Design review of the part built by this model. Coordinates are the model's own, in mm. A direction names the side the tool comes from. Round coordinates to 2 decimals unless told otherwise and drop trailing zeros. Order: outer loops, then holes, each group sorted by start corner. A loop starts at its lowest first (then second) coordinate and runs counter-clockwise, first axis right, second up. Notation, with made-up numbers: M 72,19.25 L 104,19.25 A32 ccw 104,52.25 Z; hole C 79,-3.75 d7. An arc over 180 degrees is marked long. Write each question's results on one line, items separated by ' | '. Start each with the question number.
Item 1: Clearance check with a flat-ended pin moving along its axis: pin 1 (1.3 mm diameter, centred on y = -2, z = 8.5, fed in from +X). State where the tip first meets the part, or that it passes through.
Item 2: Wall thickness on line 1 (Z direction, x = -31.6, y = -1.25); line 2 (X direction, y = -1.7, z = 10): over which ranges is each line inside the solid? List them lowest first. Write a range as [from, to].
Item 3: Take a section at A-A, the plane y = -1.27. Write out the cut boundary in (x, z), plus the area to 3 significant figures.
Item 4: The part is to be moulded in two halves that separate along Z. For faces 1 (the flat face through (-33, -2.54, 4)), 2 (the flat face through (-33, -1, 29.221)), 3 (the cylindrical face through (-31.338, -1.336, 17.025)), say which applies: +Z half, -Z half, draft (parallel to the pull), parting line (faces both ways), or undercut.
Item 5: Take a section at B-B, the plane z = -15. Write out the cut boundary in (x, y).
Item 6: Machinability: for faces 4 (the flat face through (-30.694, -1.3, 16.5)), 5 (the cylindrical face through (-31.338, -1.336, -8.375)), which of the approach directions +Z, -Z, +X, -X, +Y, -Y give a long, thin tool a straight path to every point of the face, cutting with its end or side? Answer none if there is none.
```python
from build123d import *

# Parameters (mm, degrees)
F0_W     = 2.54
F0_H     = 50.8
F1_DEPTH = 2.54
F2_R     = 0.508
F3_DEPTH = 1.27
F4_DEPTH = 1.27


with BuildPart() as f1:
    # F0 (on Front) → F1 (new body)
    with BuildSketch(Plane.XZ):
        with Locations((-33.233647, 3.821034)):
            Rectangle(F0_W, F0_H)
    extrude(amount=F1_DEPTH)

    # F2 (on face) → F3 (join)
    with BuildSketch(Plane.YZ.offset(-31.963647)):
        with Locations((-1.27, 16.521034)):
            Circle(F2_R)
        with Locations((-1.27, 3.821034)):
            Circle(F2_R)
    extrude(amount=F3_DEPTH)

    # F2 (on face) → F4 (join)
    with BuildSketch(Plane.YZ.offset(-31.963647)):
        with Locations((-1.27, -8.878966)):
            Circle(F2_R)
    extrude(amount=F4_DEPTH)


solid = f1.part
```
Results list:
1) pin 1: x = -31.96
2) line 1: [-9.39, -8.37], [3.31, 4.33], [16.01, 17.03] | line 2: [-34.5, -31.96]
3) outline: M -34.5,-21.58 L -31.96,-21.58 L -31.96,-9.39 L -30.69,-9.39 L -30.69,-8.37 L -31.96,-8.37 L -31.96,3.31 L -30.69,3.31 L -30.69,4.33 L -31.96,4.33 L -31.96,16.01 L -30.69,16.01 L -30.69,17.03 L -31.96,17.03 L -31.96,29.22 L -34.5,29.22 Z | area: 133 mm²
4) face 1: draft | face 2: +Z half | face 3: undercut
5) outline: M -34.5,-2.54 L -31.96,-2.54 L -31.96,0 L -34.5,0 Z
6) face 4: +Z, -Z, +X, +Y, -Y | face 5: +X
